```python
from build123d import *

# Parameters (mm, degrees)
F0_R     = 1.75
F1_DEPTH = 3
F0_W     = 4
F0_H     = 20.5
F0_W_2   = 19.5
F0_H_2   = 4
F2_DEPTH = 23
F3_R     = 1.75
F4_DEPTH = 28.501
F6_DEPTH = 25
F7_SIZE  = 2


with BuildPart() as f1:
    # F0 (on Top) → F1 (new body)
    with BuildSketch(Plane.XY):
        with BuildLine():
            Line((-34.3095597923, 23.5192315383), (-54.8095597923, 23.5192315383))
            Line((-54.8095597923, 23.5192315383), (-54.8095597923, 3.0192315383))
            Line((-54.8095597923, 3.0192315383), (-34.3095597923, 3.0192315383))
            Line((-34.3095597923, 3.0192315383), (-34.3095597923, 11.5921805552))
            ThreePointArc((-34.3095597923, 11.5921805552), (-35.8553848254, 11.8661100182), (-36.5595597923, 13.2692315383))
            ThreePointArc((-36.5595597923, 13.2692315383), (-35.8553848254, 14.6723530583), (-34.3095597923, 14.9462825214))
            Line((-34.3095597923, 14.9462825214), (-34.3095597923, 23.5192315383))
        make_face()
        with Locations((-44.8095597923, 13.2692315383)):
            Circle(F0_R, mode=Mode.SUBTRACT)
        with BuildLine():
            ThreePointArc((-41.5595597923, 13.2692315383), (-39.8095597923, 15.0192315383), (-38.0595597923, 13.2692315383))
            ThreePointArc((-38.0595597923, 13.2692315383), (-39.8095597923, 11.5192315383), (-41.5595597923, 13.2692315383))
        make_face(mode=Mode.SUBTRACT)
        with BuildLine():
            Line((-14.8095597923, 23.5192315383), (-34.3095597923, 23.5192315383))
            Line((-34.3095597923, 23.5192315383), (-34.3095597923, 14.9462825214))
            ThreePointArc((-34.3095597923, 14.9462825214), (-33.4064382722, 14.3150565715), (-33.0595597923, 13.2692315383))
            Line((-33.0595597923, 13.2692315383), (-31.5595597923, 13.2692315383))
            ThreePointArc((-31.5595597923, 13.2692315383), (-29.8095597923, 15.0192315383), (-28.0595597923, 13.2692315383))
            Line((-28.0595597923, 13.2692315383), (-26.5595597923, 13.2692315383))
            ThreePointArc((-26.5595597923, 13.2692315383), (-24.8095597923, 15.0192315383), (-23.0595597923, 13.2692315383))
            Line((-23.0595597923, 13.2692315383), (-21.5595597923, 13.2692315383))
            ThreePointArc((-21.5595597923, 13.2692315383), (-19.8095597923, 15.0192315383), (-18.0595597923, 13.2692315383))
            Line((-18.0595597923, 13.2692315383), (-14.8095597923, 13.2692315383))
            Line((-14.8095597923, 13.2692315383), (-14.8095597923, 23.5192315383))
        make_face()
        with BuildLine():
            Line((-34.3095597923, 11.5921805552), (-34.3095597923, 3.0192315383))
            Line((-34.3095597923, 3.0192315383), (-14.8095597923, 3.0192315383))
            Line((-14.8095597923, 3.0192315383), (-14.8095597923, 13.2692315383))
            Line((-14.8095597923, 13.2692315383), (-18.0595597923, 13.2692315383))
            ThreePointArc((-18.0595597923, 13.2692315383), (-19.8095597923, 11.5192315383), (-21.5595597923, 13.2692315383))
            Line((-21.5595597923, 13.2692315383), (-23.0595597923, 13.2692315383))
            ThreePointArc((-23.0595597923, 13.2692315383), (-24.8095597923, 11.5192315383), (-26.5595597923, 13.2692315383))
            Line((-26.5595597923, 13.2692315383), (-28.0595597923, 13.2692315383))
            ThreePointArc((-28.0595597923, 13.2692315383), (-29.8095597923, 11.5192315383), (-31.5595597923, 13.2692315383))
            Line((-31.5595597923, 13.2692315383), (-33.0595597923, 13.2692315383))
            ThreePointArc((-33.0595597923, 13.2692315383), (-33.4064382722, 12.2234065051), (-34.3095597923, 11.5921805552))
        make_face()
    extrude(amount=F1_DEPTH)

    # F0 (on Top) → F2 (join)
    with BuildSketch(Plane.XY):
        with Locations((-56.8095597923, 13.2692315383)):
            Rectangle(F0_W, F0_H)
        with Locations((-24.5595597923, 1.0192315383)):
            Rectangle(F0_W_2, F0_H_2)
        with Locations((-24.5595597923, 25.5192315383)):
            Rectangle(F0_W_2, F0_H_2)
    extrude(amount=F2_DEPTH)

    # F3 (on face) → F4 (cut, through all)
    with BuildSketch(Plane(origin=(0, 27.5192315383, 0), x_dir=(-1, 0, 0), z_dir=(0, 1, 0))):
        with Locations((19.8095597923, 13)):
            Circle(F3_R)
        with Locations((24.8095597923, 13)):
            Circle(F3_R)
        with Locations((29.8095597923, 13)):
            Circle(F3_R)
        with Locations((39.8095597923, 13)):
            Circle(F3_R)
        with Locations((44.8095597923, 13)):
            Circle(F3_R)
        with Locations((49.8095597923, 13)):
            Circle(F3_R)
    extrude(amount=-F4_DEPTH, mode=Mode.SUBTRACT)

    # F5 (on face) → F6 (cut)
    with BuildSketch(Plane(origin=(-58.8095597923, 0, 0), x_dir=(0, -1, 0), z_dir=(-1, 0, 0))):
        with BuildLine():
            Line((-13.0192315383, 13), (-11.7817946712, 14.2374368671))
            ThreePointArc((-11.7817946712, 14.2374368671), (-13.0192315383, 14.75), (-14.2566684054, 14.2374368671))
            Line((-14.2566684054, 14.2374368671), (-13.0192315383, 13))
        make_face()
        with BuildLine():
            ThreePointArc((-14.2566684054, 11.7625631329), (-13.0192315383, 11.25), (-11.7817946712, 11.7625631329))
            Line((-11.7817946712, 11.7625631329), (-13.0192315383, 13))
            Line((-13.0192315383, 13), (-14.2566684054, 11.7625631329))
        make_face()
        with BuildLine():
            ThreePointArc((-11.2692315383, 13), (-11.4024423564, 13.6696960066), (-11.7817946712, 14.2374368671))
            Line((-11.7817946712, 14.2374368671), (-13.0192315383, 13))
            Line((-13.0192315383, 13), (-11.7817946712, 11.7625631329))
            ThreePointArc((-11.7817946712, 11.7625631329), (-11.4024423564, 12.3303039934), (-11.2692315383, 13))
        make_face()
        with BuildLine():
            Line((-13.0192315383, 13), (-14.2566684054, 14.2374368671))
            ThreePointArc((-14.2566684054, 14.2374368671), (-14.7692315383, 13), (-14.2566684054, 11.7625631329))
            Line((-14.2566684054, 11.7625631329), (-13.0192315383, 13))
        make_face()
    extrude(amount=-F6_DEPTH, mode=Mode.SUBTRACT)

    # F7
    f7_edges = [f1.edges().sort_by_distance(p)[0] for p in [
        (-24.55956, -0.980768, 23),
        (-14.80956, -0.980768, 11.5),
        (-24.55956, -0.980768, 0),
        (-14.80956, 13.269232, 0),
        (-14.80956, 27.519232, 11.5),
        (-14.80956, 1.019232, 23),
        (-14.80956, 25.519232, 23),
        (-24.55956, 27.519232, 23),
        (-34.30956, 25.519232, 23),
        (-34.30956, 1.019232, 23),
        (-24.55956, 27.519232, 0),
        (-58.80956, 23.519232, 11.5),
        (-58.80956, 3.019232, 11.5),
        (-58.80956, 13.269232, 23),
        (-58.80956, 13.269232, 0),
    ]]
    chamfer(f7_edges, length=F7_SIZE)


solid = f1.part
```
Work out the finished part from the listing and answer in its coordinate system (mm). A direction names the side the tool comes from. Coordinates: 2 decimals unless noted, no trailing zeros. Write each loop counter-clockwise with the first axis right and the second up, starting at its lowest first coordinate (ties: lowest second). Pieces come first, ordered by that corner, then holes. Notation, with made-up numbers: (-18.75, -3.75) - (6.25, -3.75) arc R25 cw to (6.25, 33.25) - close; hole circle Ø2 at (29.25, 80.25). An arc over 180 degrees is marked (long way). Answer as a JSON object with one key per item and string values.
Q1. Find section A-A (z = 15.5). Write down the section's boundary in (x, y), plus the area to 3 significant figures.
Results list:
{"outline": "(-58.81, 5.02) - (-56.81, 3.02) - (-54.81, 3.02) - (-54.81, 23.52) - (-56.81, 23.52) - (-58.81, 21.52) - close; (-34.31, -0.98) - (-16.81, -0.98) - (-14.81, 1.02) - (-14.81, 3.02) - (-34.31, 3.02) - close; (-34.31, 23.52) - (-14.81, 23.52) - (-14.81, 25.52) - (-16.81, 27.52) - (-34.31, 27.52) - close", "area": "230 mm^2"}
Q2. Find section D-D (y = 6.75). Write down the section's boundary in (x, z).
Results list:
{"outline": "(-58.81, 2) - (-56.81, 0) - (-16.81, 0) - (-14.81, 2) - (-14.81, 3) - (-54.81, 3) - (-54.81, 23) - (-56.81, 23) - (-58.81, 21) - close"}
Q3. For a pull along Z with two mould halves and no side action, classify faces 4 (the flat face through (-15.82, 24.51, 22.01)), 5 (the flat face through (-58.81, 15, 11)), 6 (the cylindrical face through (-28.52, 1.047, 14.183)) as pulls with the +Z half, pulls with the -Z half, needs draft (parallel to the pull), parting line crosses it, or undercut.
Results list:
{"face 4": "pulls with the +Z half", "face 5": "needs draft", "face 6": "undercut"}
Q4. Find section C-C (x = -40.5). Write down the section's boundary in (y, z), plus the area to 3 significant figures.
Results list:
{"outline": "(3.02, 0) - (11.66, 0) - (11.66, 3) - (3.02, 3) - close; (14.88, 0) - (23.52, 0) - (23.52, 3) - (14.88, 3) - close", "area": "51.9 mm^2"}
Q5. Find section B-B (y = 2.5). Write down the section's boundary in (x, z).
Results list:
{"outline": "(-34.31, 0) - (-16.81, 0) - (-14.81, 2) - (-14.81, 21) - (-16.81, 23) - (-32.31, 23) - (-34.31, 21) - close; hole circle Ø3.5 at (-29.81, 13); hole circle Ø3.5 at (-24.81, 13); hole circle Ø3.5 at (-19.81, 13)"}
Q6. Given pin 1 Ø4.5 at (x, y) = (-19.81, 13.27) entering from +Z; pin 2 Ø6 at (y, z) = (16.5, 11.5) entering from +X, each flat-ended and moving along its own axis, determine where each tip first touches the part or whether it passes through.
Results list:
{"pin 1": "stops at z = 3", "pin 2": "stops at x = -54.81"}
Q7. Which of the six approach directions +Z, -Z, +X, -X, +Y, -Y give full straight-line access (tool end or side, diameter ignored) to faces 1 (the flat face through (-54.81, 13, 11)), 2 (the flat face through (-22.5, 23.519, 12.9)), 3 (the flat face through (-25.68, 26.53, 1.01))?
Results list:
{"face 1": "+Z, +X, +Y, -Y", "face 2": "+Z, +X", "face 3": "-Z, +X, -X, +Y"}
Q8. Consider L1, parallel to Y at x = -26, z = 4; L2, parallel to X at y = 6, z = 15.5; L3, parallel to Z at x = -54, y = 6. Determine where each line is inside the solid, lowest interval first. Write a range as from..to.
Results list:
{"L1": "y = -0.98..3.02, 23.52..27.52", "L2": "x = -58.81..-54.81", "L3": "z = 0..3"}
